Input: dimensioned drawing with shaded views. Units: mm. Origin: part minimum x, y, z. A direction names the side the tool comes from. Coordinates: 2 decimals unless noted, no trailing zeros. Loops run counter-clockwise (first coordinate to the right, second up) from the corner with the lowest first, then second, coordinate; pieces in that order, holes last.
(1) Mould query, pull axis X, two halves, no side actions, for the marked faces 3, 4 and 5. Classes: released by +X, released by -X, zero draft, split by the parting line, or undercut.
(2) Line query: L1, parallel to Y at x = 45.5, z = 8.5; L2, parallel to X at y = 75.5, z = 4; L3, parallel to X at y = 38, z = 5. Output: solid intervals per line, ascending.
(3) Section B-B, the plane y = 38. Return loops of the section in (x, z) (3 decimals), then the cut area to 3 significant figures.
(4) Contact query for flat-ended pins moving along their axis: P1, Ø12, axis at x = 43.5, z = 7.5, coming from the +Y side; P2, Ø10, axis at y = 49, z = 11, coming from the -X side; P3, Ø4, axis at y = 49.5, z = 27, coming from the +X side; P4, Ø8, axis at x = 24, z = 13, coming from the -Y side. Output: stop coordinate, or through.
(5) Section C-C, the plane x = 57.5. Return loops of the section in (y, z).
(6) Set-up query: the marked faces 1 and 2. Return all of +Z, -Z, +X, -X, +Y, -Y with unobstructed straight access to the full face (end or side cutting, diameter ignored); none if empty.
(7) Section A-A, the plane z = 13. Return loops of the section in (x, y).
(8) Section D-D, the plane z = 24.5. Return loops of the section in (x, y), then the cut area to 3 significant figures.
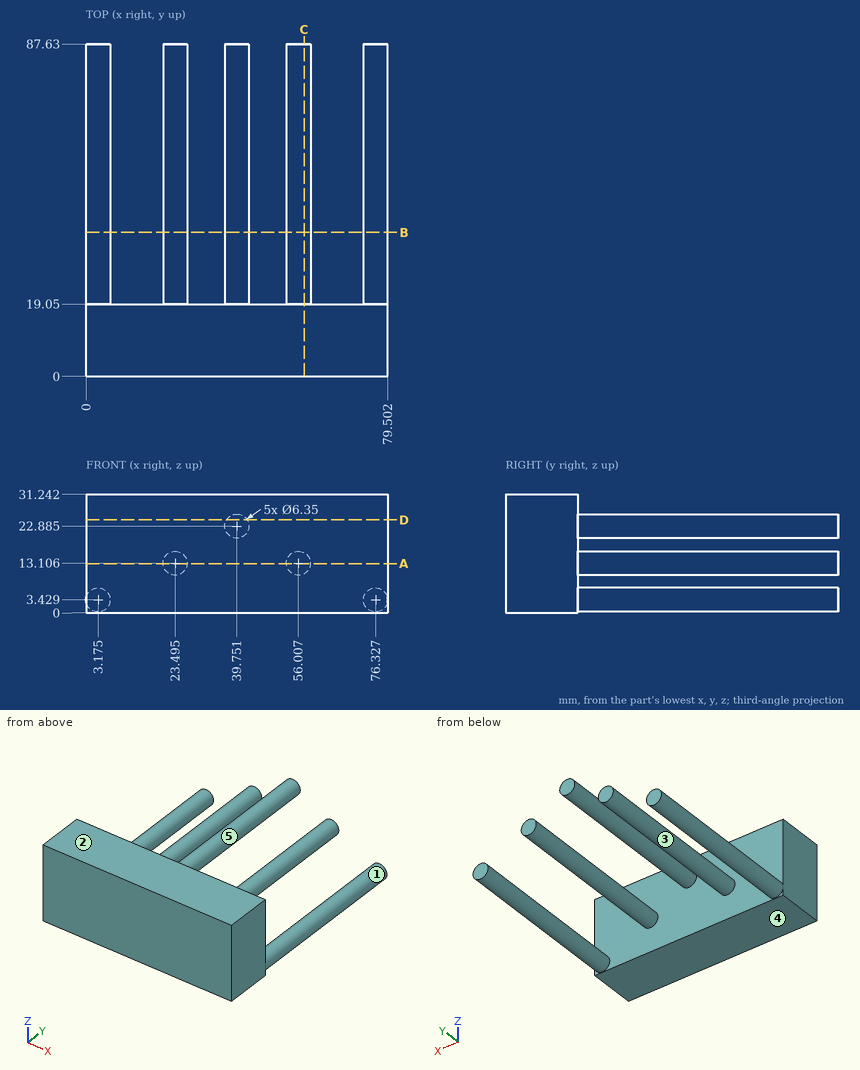
Report:
1. face 3: undercut
1. face 4: zero draft
1. face 5: split by the parting line
2. L1: y = 0 to 19.05
2. L2: x = 0.05 to 6.3, 73.2 to 79.45
2. L3: x = 0.42 to 5.93, 73.57 to 79.09
3. outline: circle Ø6.35 at (3.175, 3.429); circle Ø6.35 at (23.495, 13.106); circle Ø6.35 at (39.751, 22.885); circle Ø6.35 at (56.007, 13.106); circle Ø6.35 at (76.327, 3.429)
3. area: 158 mm2
4. P1: stops at y = 19.05
4. P2: stops at x = 1.31
4. P3: stops at x = 42.12
4. P4: stops at y = 0
5. outline: (0, 0) - (19.05, 0) - (19.05, 10.3) - (87.63, 10.3) - (87.63, 15.91) - (19.05, 15.91) - (19.05, 31.24) - (0, 31.24) - close
6. face 1: +Y
6. face 2: +Z, +X, -X, +Y, -Y
7. outline: (0, 0) - (79.5, 0) - (79.5, 19.05) - (59.18, 19.05) - (59.18, 87.63) - (52.83, 87.63) - (52.83, 19.05) - (26.67, 19.05) - (26.67, 87.63) - (20.32, 87.63) - (20.32, 19.05) - (0, 19.05) - close
8. outline: (0, 0) - (79.5, 0) - (79.5, 19.05) - (42.48, 19.05) - (42.48, 87.63) - (37.02, 87.63) - (37.02, 19.05) - (0, 19.05) - close
8. area: 1,890 mm2
